```python
from build123d import *

# Parameters (mm, degrees)
F1_DEPTH = 457.2
F2_DEPTH = 50.8
F4_DEPTH = 35.922024


with BuildPart() as f1:
    # F0 (on Top) → F1 (new body)
    with BuildSketch(Plane.XY):
        Polygon((-12.7, 12.7), (0, 0), (0, 50.8), (-12.7, 50.8), align=None)
    extrude(amount=F1_DEPTH)

    # F1_face (on face) → F2 (cut)
    with BuildSketch(Plane(origin=(-6.047619, 28.42381, 0), x_dir=(1, 0, 0), z_dir=(0, 0, -1))):
        Polygon((6.047619, 28.42381), (-6.652381, 15.72381), (-6.652381, -22.37619), (6.047619, -22.37619), align=None)
        Polygon((-6.652381, 15.72381), (6.047619, 28.42381), (6.047619, -22.37619), (-6.652381, -22.37619), align=None)
    extrude(amount=-F2_DEPTH, mode=Mode.SUBTRACT)

    # F3 (on face) → F4 (cut, through all)
    with BuildSketch(Plane(origin=(0, 0, 0), x_dir=(0.707107, -0.707107, 0), z_dir=(-0.707107, -0.707107, 0))):
        Polygon((3.225248, 381), (0, 381), (-25.4, 381), (-25.4, 376.2375), (0, 376.2375), (3.225248, 376.2375), align=None)
        Polygon((5.052605, 300.0375), (0, 300.0375), (-25.4, 300.0375), (-25.4, 295.275), (5.052605, 295.275), align=None)
        Polygon((-25.4, 207.9625), (0, 207.9625), (8.918187, 207.9625), (8.918187, 212.725), (-25.4, 212.725), align=None)
        Polygon((-25.4, 127), (0, 127), (10.666735, 127), (10.666735, 131.7625), (0, 131.7625), (-25.4, 131.7625), align=None)
    extrude(amount=-F4_DEPTH, mode=Mode.SUBTRACT)


solid = f1.part
```
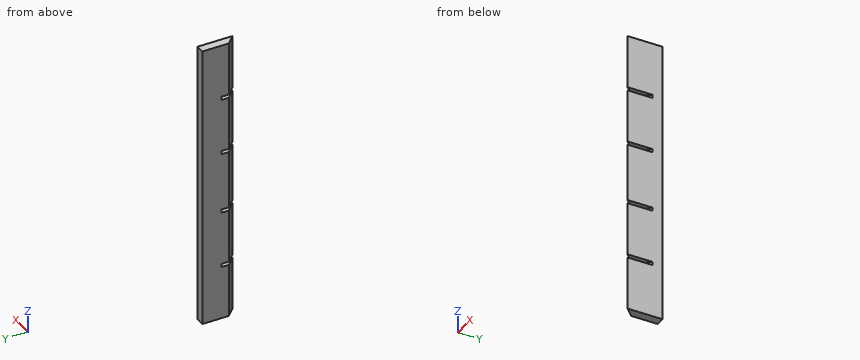
Can you work these out from the model? Positions are in its coordinate system, mm. Coordinates: 2 decimals unless noted, no trailing zeros. Loops run counter-clockwise (first coordinate to the right, second up) from the corner with the lowest first, then second, coordinate; pieces in that order, holes last. Notation, with made-up numbers: (23, -25) - (36, -25) arc R22 ccw to (36, 11) - close; hole circle Ø4 at (-25, 87.5). An arc over 180 degrees is marked (long way). Use a Markdown table: item, result.
Item 1: If I drill on probe 1 along Z at (x, y) = (-5, 25.5) (1 decimal); probe 2 along X at (y, z) = (6, 346.5); probe 3 along Y at (x, z) = (-5.75, 285), over which ranges is the centre line in solid material (lowest first)? Write a range as from..to.
Numbers:
| item | result |
|---|---|
| probe 1 | z = 50.8..127, 131.8..208, 212.7..295.3, 300..376.2, 381..457.2 |
| probe 2 | x = -6..0 |
| probe 3 | y = 5.75..50.8 |
Item 2: I want a section at A-A on y = 5. Please give me the cut outline in (x, z) (1 decimal).
Numbers:
| item | result |
|---|---|
| outline | (-5, 50.8) - (0, 50.8) - (0, 127) - (-5, 127) - close; (-5, 131.8) - (0, 131.8) - (0, 208) - (-5, 208) - close; (-5, 212.7) - (0, 212.7) - (0, 295.3) - (-5, 295.3) - close; (-5, 300) - (0, 300) - (0, 376.2) - (-5, 376.2) - close; (-5, 381) - (0, 381) - (0, 457.2) - (-5, 457.2) - close |
Item 3: I want a section at B-B on x = -3.5. Please give me the cut outline in (y, z) (1 decimal), and give its area (3 significant figures).
Numbers:
| item | result |
|---|---|
| outline | (3.5, 50.8) - (50.8, 50.8) - (50.8, 457.2) - (3.5, 457.2) - (3.5, 381) - (32.4, 381) - (32.4, 376.2) - (3.5, 376.2) - (3.5, 300) - (32.4, 300) - (32.4, 295.3) - (3.5, 295.3) - (3.5, 212.7) - (32.4, 212.7) - (32.4, 208) - (3.5, 208) - (3.5, 131.8) - (32.4, 131.8) - (32.4, 127) - (3.5, 127) - close |
| area | 18,700 mm2 |
Item 4: Will these pins go through, and if not, where does the flat tip stop? pin 1 (1 mm diameter, centred on x = -4, z = 101.5, fed in from -Y); pin 2 (5 mm diameter, centred on x = -8, z = 402, fed in from -Y).
Numbers:
| item | result |
|---|---|
| pin 1 | stops at y = 3.5 |
| pin 2 | stops at y = 5.5 |
Item 5: I want a section at C-C on z = 231.5. Please give me the cut outline in (x, y).
Numbers:
| item | result |
|---|---|
| outline | (-12.7, 12.7) - (0, 0) - (0, 50.8) - (-12.7, 50.8) - close |
